Here's the drawing with two shaded views (mm, measured from the low corner). I have some questions. A direction names the side the tool comes from. Give positions to 0.01 mm unless a question says otherwise; leave off trailing zeros. Loops run counter-clockwise (first coordinate to the right, second up) from the corner with the lowest first, then second, coordinate; pieces in that order, holes last. Notation, with made-up numbers: M -19,-37.75 L 9,-37.75 A20 ccw 9,0.25 Z; hole C -6.75,28 d10. An arc over 180 degrees is marked long. Use a Markdown table: item, result. Add a question column.
1) Suppose I cut it at B-B on y = 16.25. List the corners of the cut face in (x, z) for me.
2) We'd pull the mould along Y, two halves only. Please class the marked faces 1, 2, 3 and 4: +Y half, -Y half, draft (parallel to the pull), parting line (faces both ways), or undercut.
3) Which directions (+Z, -Z, +X, -X, +Y, -Y) give clear straight access to the entire face, cutting with the end or side of a thin tool? Please do the marked faces 5 and 6.
4) Will these pins go through, and if not, where does the flat tip stop? pin 1 Ø1.9 at (x, y) = (2.5, 41) entering from +Z; pin 2 Ø1.2 at (y, z) = (28, 8.5) entering from +X.
5) Suppose I cut it at A-A on z = 22.5. List the corners of the cut face in (x, y) for me (3 decimals), and give its area (3 significant figures).
6) Suppose I cut it at D-D on x = 2.5. List the corners of the cut face in (y, z) for me (3 decimals), and give its area (3 significant figures).
7) Suppose I cut it at C-C on z = 11. List the corners of the cut face in (x, y) for me, and give its area (3 significant figures).
8) If I drill on line 1 along Y through (x, z) = (0.7, 4.75); line 2 along Z through (x, y) = (1.1, 27.75); line 3 along Y through (x, z) = (2.5, 21.75) (3 decimals), over which ranges is the centre line in solid material (lowest first)? Write a range as [from, to].
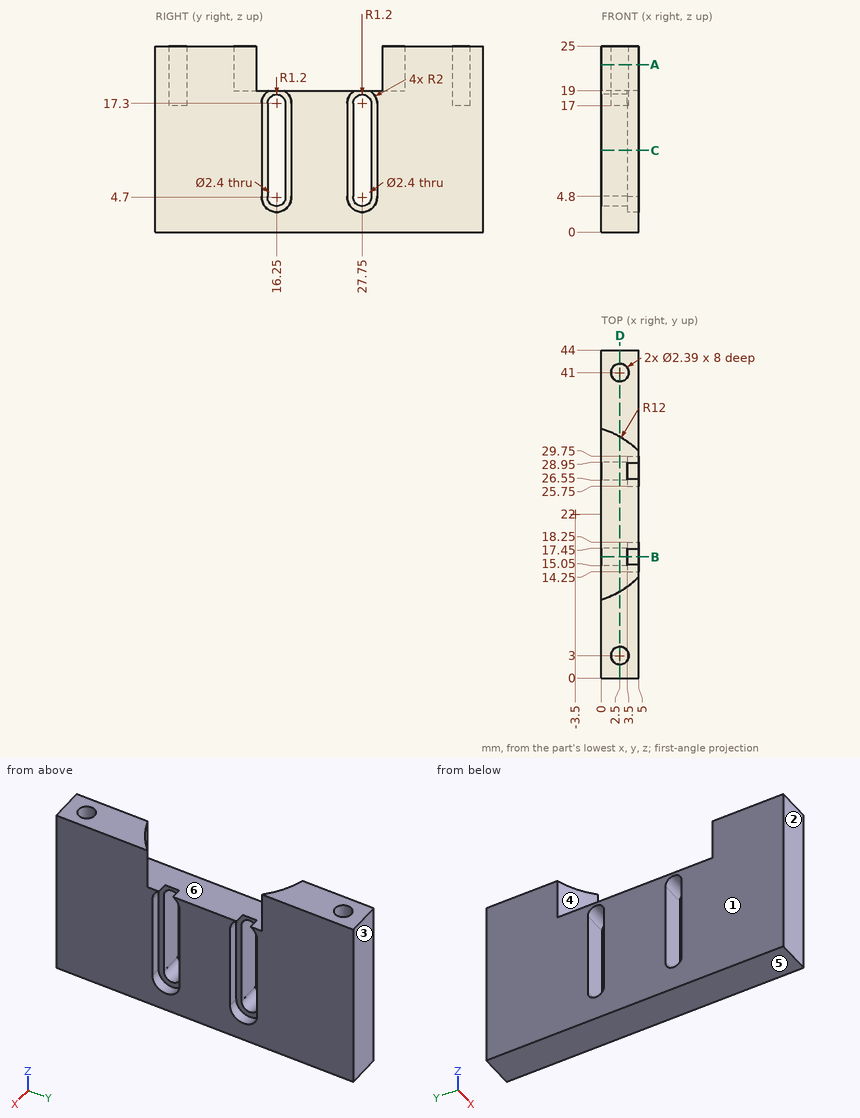
Answer block:
| question | item | result |
|---|---|---|
| 1 | outline | M 0,0 L 5,0 L 5,2.7 L 3.5,2.7 L 3.5,3.5 L 0,3.5 Z; M 0,18.5 L 3.5,18.5 L 3.5,19 L 0,19 Z |
| 2 | face 1 | draft |
| 2 | face 2 | -Y half |
| 2 | face 3 | +Y half |
| 2 | face 4 | undercut |
| 3 | face 5 | -Z, +X, -X, +Y, -Y |
| 3 | face 6 | +Z, -X |
| 4 | pin 1 | stops at z = 17 |
| 4 | pin 2 | passes through |
| 5 | outline | M 0,0 L 5,0 L 5,13.529 A12 cw 0,10.522 Z; M 0,33.478 A12 cw 5,30.471 L 5,44 L 0,44 Z; hole C 2.5,3 d2.39; hole C 2.5,41 d2.39 |
| 5 | area | 108 mm^2 |
| 6 | outline | M 0,0 L 44,0 L 44,25 L 42.195,25 L 42.195,17 L 39.805,17 L 39.805,25 L 32.392,25 L 32.392,19 L 11.608,19 L 11.608,25 L 4.195,25 L 4.195,17 L 1.805,17 L 1.805,25 L 0,25 Z; hole M 15.05,4.8 L 15.054,4.8 A1.2 ccw long 17.446,4.8 L 17.45,4.8 L 17.45,17.3 A1.2 ccw 15.05,17.3 Z; hole M 26.55,4.8 L 26.554,4.8 A1.2 ccw long 28.946,4.8 L 28.95,4.8 L 28.95,17.3 A1.2 ccw 26.55,17.3 Z |
| 6 | area | 868 mm^2 |
| 7 | outline | M 0,0 L 5,0 L 5,14.25 L 3.5,14.25 L 3.5,15.05 L 0,15.05 Z; M 0,17.45 L 3.5,17.45 L 3.5,18.25 L 5,18.25 L 5,25.75 L 3.5,25.75 L 3.5,26.55 L 0,26.55 Z; M 0,28.95 L 3.5,28.95 L 3.5,29.75 L 5,29.75 L 5,44 L 0,44 Z |
| 7 | area | 191 mm^2 |
| 8 | line 1 | y = [0, 15.05], [17.45, 26.55], [28.95, 44] |
| 8 | line 2 | z = [0, 3.5], [18.5, 19] |
| 8 | line 3 | y = [0, 1.805], [4.195, 11.608], [32.392, 39.805], [42.195, 44] |
